from build123d import *

# Parameters (mm, degrees)
SKETCH1_W           = 80
SKETCH1_H           = 65.45
BOSS_EXTRUDE1_DEPTH = 31
BOSS_EXTRUDE3_DEPTH = 5
CHAMFER2_SIZE       = 25
CHAMFER2_SIZE2      = 20.977490779
SHELL2_START        = -36
SHELL2_DEPTH        = 72
SHELL2_START_2      = -41
SHELL2_2_OUTLINE_W  = 1
SHELL2_2_OUTLINE_H  = 57.45
SHELL2_2_DEPTH      = 82
SKETCH6_R           = 4.86874318
CUT_EXTRUDE1_DEPTH  = 5
BOSS_EXTRUDE4_DEPTH = 8
BOSS_EXTRUDE5_REACH = 107.939
BOSS_EXTRUDE5_START = 29.5
SKETCH10_W          = 12.25
SKETCH10_H          = 9
CUT_EXTRUDE2_DEPTH  = 6
CHAMFER3_SIZE       = 2
CHAMFER3_SIZE2      = 1.865030172
CHAMFER4_SIZE       = 7.098078142
CHAMFER4_SIZE_2     = 10
CHAMFER5_SIZE       = 10
CHAMFER7_SIZE       = 5
SKETCH11_R          = 0.93
CUT_EXTRUDE3_DEPTH  = 7


# Read off the part's stored shape, not the designer's step: Shell2
with BuildPart() as part:
    # Sketch1 → Boss-Extrude1 (new body)
    with BuildSketch(Plane(origin=(0, 0, 0), x_dir=(1, 0, 0), z_dir=(0, 1, 0))):
        Rectangle(SKETCH1_W, SKETCH1_H)
    extrude(amount=BOSS_EXTRUDE1_DEPTH)

    # Sketch5 → Boss-Extrude3 (add)
    with BuildSketch(Plane.ZY.offset(40)):
        Polygon((-32.725, 31), (-20.625, 31), (8.005, 31), (32.725, 31), (32.725, 26), (2.6203214, 26), (6.0203214, 22.6), (-5.2796786, 22.6), (-1.8796786, 26), (-16.125, 26), (-12.725, 22.6), (-24.025, 22.6), (-20.625, 26), (-32.725, 26), align=None)
    boss_extrude3 = extrude(amount=BOSS_EXTRUDE3_DEPTH)

    # Mirror1: Boss-Extrude3 across plane
    add(boss_extrude3.mirror(Plane(origin=(0, 0, 0), x_dir=(0, 0, 1), z_dir=(1, 0, 0))))

    # Chamfer2
    chamfer2_edges = [part.edges().sort_by_distance(p)[0] for p in [
        (0, 0, 32.725),
    ]]
    chamfer2_side = [part.faces().sort_by_distance(p)[0] for p in [
        (0, 0, 0),
    ]]
    chamfer(chamfer2_edges, length=CHAMFER2_SIZE, length2=CHAMFER2_SIZE2, reference=chamfer2_side[0])

    # Shell2 outline → Shell2 (cut)
    with BuildSketch(Plane.YZ.offset(SHELL2_START)):
        Polygon((22.842721412, 28.725), (4, 6.269119063), (4, -28.725), (31, -28.725), (31, 28.725), align=None)
    extrude(amount=SHELL2_DEPTH, mode=Mode.SUBTRACT)

    # Shell2 2 outline → Shell2 2 (cut)
    with BuildSketch(Plane.YZ.offset(SHELL2_START_2)):
        with Locations((30.5, 0)):
            Rectangle(SHELL2_2_OUTLINE_W, SHELL2_2_OUTLINE_H)
    extrude(amount=SHELL2_2_DEPTH, mode=Mode.SUBTRACT)

    # Sketch6 → Cut-Extrude1 (cut)
    with BuildSketch(Plane(origin=(0, 4, 24.632603001), x_dir=(1, 0, 0), z_dir=(0, 1, 0))):
        with Locations(Location((22, 23.453346141, 0), (0, 0, 270))):
            Circle(SKETCH6_R)
        with Locations(Location((-22, 23.453346141, 0), (0, 0, 270))):
            Circle(SKETCH6_R)
    extrude(amount=-CUT_EXTRUDE1_DEPTH, mode=Mode.SUBTRACT)

    # Sketch7 → Boss-Extrude4 (add)
    with BuildSketch(Plane.XY.offset(-28.725)):
        Polygon((-14.5, 13.5), (14.5, 13.5), (14.5, 28.31455183), (13.5, 28.31455183), (13.5, 14.706896552), (-13.5, 14.706896552), (-13.5, 28.31455183), (-14.5, 28.31455183), align=None)
    extrude(amount=BOSS_EXTRUDE4_DEPTH)

    # Sketch8 → Boss-Extrude5 (add, up to next)
    with BuildSketch(Plane.XY.offset(-20.725).offset(BOSS_EXTRUDE5_START), mode=Mode.PRIVATE) as boss_extrude5_sk1:
        Polygon((-13.5, 14.706896552), (-13.5, 28.31455183), (-14.5, 28.31455183), (-14.5, 14.706896552), (-14.5, 13.5), (-13.5, 13.5), (13.5, 13.5), (14.5, 13.5), (14.5, 14.706896552), (14.5, 28.31455183), (13.5, 28.31455183), (13.5, 14.706896552), align=None)
    boss_extrude5_tool1 = extrude(boss_extrude5_sk1.sketch, amount=BOSS_EXTRUDE5_REACH, mode=Mode.PRIVATE) - part.part
    add(boss_extrude5_tool1.solids().sort_by_distance((-14.174351, 21.510724, 8.775))[0])

    # Sketch10 → Cut-Extrude2 (cut)
    with BuildSketch(Plane.XZ):
        with Locations((-26.125, -23.025)):
            Rectangle(SKETCH10_W, SKETCH10_H)
        with Locations((26.125, -23.025)):
            Rectangle(SKETCH10_W, SKETCH10_H)
    extrude(amount=-CUT_EXTRUDE2_DEPTH, mode=Mode.SUBTRACT)

    # Chamfer3
    chamfer3_edges = [part.edges().sort_by_distance(p)[0] for p in [
        (0, 31, -32.725),
    ]]
    chamfer3_side = [part.faces().sort_by_distance(p)[0] for p in [
        (0, 15.756916996, -32.725),
    ]]
    chamfer(chamfer3_edges, length=CHAMFER3_SIZE, length2=CHAMFER3_SIZE2, reference=chamfer3_side[0])

    # Chamfer4
    # the kernel refuses this chamfer: 10, 7.098078142 mm, written as the material it adds along each edge
    with BuildSketch(Plane(origin=(14.5, 13.5, 17.590778193), x_dir=(0, -0.6849156240265527, -0.728622390518105), z_dir=(-1, 0, 0))) as chamfer4_piece_1_section:
        Polygon((CHAMFER4_SIZE * 0.998412410217, -CHAMFER4_SIZE * 0.0563263630269), (CHAMFER4_SIZE_2 * 0.728622390518, -CHAMFER4_SIZE_2 * 0.684915624027), (0, 0), align=None)
    chamfer4_piece_1 = extrude(amount=29, mode=Mode.PRIVATE)
    chamfer4_piece_1 = split(chamfer4_piece_1, bisect_by=Plane(origin=(0, 11.943437141, 8.775), z_dir=(0, 0, 1)), keep=Keep.TOP, mode=Mode.PRIVATE)
    add(chamfer4_piece_1)

    # Chamfer5
    # the kernel refuses this chamfer: 10 mm, written as the material it adds along each edge
    with BuildSketch(Plane(origin=(-14.5, 13.5, -28.725), x_dir=(0, -0.9996219169112968, -0.02749587661058701), z_dir=(1, 0, 0))) as chamfer5_piece_1_section:
        Polygon((CHAMFER5_SIZE * 0.999621916911, -CHAMFER5_SIZE * 0.0274958766106), (-CHAMFER5_SIZE * 0.0274958766106, -CHAMFER5_SIZE * 0.999621916911), (0, 0), align=None)
    chamfer5_piece_1 = extrude(amount=29, mode=Mode.PRIVATE)
    chamfer5_piece_1 = split(chamfer5_piece_1, bisect_by=Plane(origin=(0, 10.042815877, -20.725), z_dir=(0, 0, -1)), keep=Keep.TOP, mode=Mode.PRIVATE)
    add(chamfer5_piece_1)

    # Chamfer7
    chamfer7_edges = [part.edges().sort_by_distance(p)[0] for p in [
        (40, 10.48874539, 20.225),
        (-40, 10.48874539, 20.225),
        (-40, 13, -32.725),
        (40, 13, -32.725),
    ]]
    chamfer(chamfer7_edges, length=CHAMFER7_SIZE)

    # Sketch11 → Cut-Extrude3 (cut)
    with BuildSketch(Plane(origin=(0, 30, 0), x_dir=(1, 0, 0), z_dir=(0, 1, 0))):
        with Locations(Location((38.849613738, -26.574613738, 0), (0, 0, 270))):
            Circle(SKETCH11_R)
        with Locations(Location((38.849613738, 26.574613738, 0), (0, 0, 90))):
            Circle(SKETCH11_R)
        with Locations(Location((-38.849613738, 26.574613738, 0), (0, 0, 270))):
            Circle(SKETCH11_R)
        with Locations(Location((-38.849613738, -26.574613738, 0), (0, 0, 90))):
            Circle(SKETCH11_R)
    extrude(amount=-CUT_EXTRUDE3_DEPTH, mode=Mode.SUBTRACT)


solid = part.part
Geometry: final body of the model. Coordinates: model frame, mm. A direction names the side the tool comes from. Round coordinates to 2 decimals unless told otherwise and drop trailing zeros. Loops run counter-clockwise (first coordinate to the right, second up) from the corner with the lowest first, then second, coordinate; pieces in that order, holes last. Notation, with made-up numbers: (14.25, -22.75) - (32.25, -22.75) arc R36 ccw to (32.25, 12.25) - close; hole circle Ø5 at (65, 72). An arc over 180 degrees is marked (long way). Write each question's results on one line, items separated by ' | '. Start each with the question number.
1) Cut plane C-C on z = -9. Return loops of the section in (x, y), then the cut area to 3 significant figures.
2) First-contact query: P1, Ø8, axis at x = 22, z = 1.18, coming from the -Y side; P2, Ø4, axis at y = 11, z = 0, coming from the +X side; P3, Ø10, axis at y = 16, z = 16, coming from the -X side; P4, Ø0.5, axis at x = 14, z = -26, coming from the +Y side. Flat tips, straight axial feed; report the tip coordinate or a pass-through.
3) Line query: probe 1 along X at (y, z) = (21, 25); probe 2 along X at (y, z) = (26, 1); probe 3 along X at (y, z) = (8, -28) (3 decimals). Output: solid intervals per line, ascending. Write a range as [from, to].
4) Mould query, pull axis Y, two halves, no side actions, for faces 1 (the face through (-42.465, 24.324, -14.449)), 2 (the face through (-1, 0, -13)), 3 (the face through (45, 28, 0)). Classes: released by +Y, released by -Y, zero draft, split by the parting line, or undercut.
5) Cut plane B-B on x = 8. Return loops of the section in (y, z) (1 decimal).
6) Access query for faces 4 (the face through (38.809, 26.549, -25.646)), 5 (the face through (26, 2, -27.525)), 6 (the face through (-42, 22.6, 0)), 7 (the face through (-0.203, 7.698, -24.528)). Directions: +Z, -Z, +X, -X, +Y, -Y. A direction counts if a zero-diameter tool reaches every point of the face in a straight line with its end or side. Return the directions, or none.
7) Cut plane D-D on y = 16. Return loops of the section in (x, z) (3 decimals), then the cut area to 3 significant figures.
8) Cut plane A-A on x = 22. Count the separate pieces of the cut face and the enclosed holes in it, then the cut area to 3 significant figures.
Verdict:
1) outline: (-45, 26) - (-40, 26) - (-40, 0) - (40, 0) - (40, 26) - (45, 26) - (45, 31) - (41, 31) - (41, 30) - (36, 30) - (36, 4) - (-36, 4) - (-36, 30) - (-41, 30) - (-41, 31) - (-45, 31) - close | area: 576 mm2
2) P1: passes through | P2: stops at x = 40 | P3: stops at x = -40 | P4: stops at y = 28.31
3) probe 1: x = [-39.98, -36], [-14.5, -13.5], [13.5, 14.5], [36, 39.98] | probe 2: x = [-45, -36], [36, 45] | probe 3: x = [-39.725, -36], [-14.5, 14.5], [36, 39.725]
4) face 1: undercut | face 2: released by -Y | face 3: zero draft
5) outline: (0, -32.7) - (29, -32.7) - (31, -30.9) - (31, -28.7) - (14.7, -28.7) - (14.7, -20.7) - (11.5, -20.7) - (4, -28.2) - (4, 6.3) - (8.9, 12.2) - (12.3, 8.8) - (14.7, 8.8) - (14.7, 19) - (22.8, 28.7) - (31, 28.7) - (31, 32.7) - (21, 32.7) - (0, 7.7) - close
6) face 4: +Y | face 5: +Y, -Y | face 6: +Z, -Z, -X, -Y | face 7: none
7) outline: (-40, -27.725) - (-35, -32.725) - (35, -32.725) - (40, -27.725) - (40, 19.014) - (35, 26.793) - (-35, 26.793) - (-40, 19.014) - close; hole (-36, -28.725) - (-14.5, -28.725) - (-14.5, -20.725) - (-13.5, -20.725) - (-13.5, -28.725) - (13.5, -28.725) - (13.5, -20.725) - (14.5, -20.725) - (14.5, -28.725) - (36, -28.725) - (36, 20.57) - (14.5, 20.57) - (14.5, 8.775) - (13.5, 8.775) - (13.5, 20.57) - (-13.5, 20.57) - (-13.5, 8.775) - (-14.5, 8.775) - (-14.5, 20.57) - (-36, 20.57) - close | area: 1,190 mm2
8) separate pieces: 3 | enclosed holes: 0 | area: 350 mm2
